Autodesk Inventor part; units mm, degrees
ref_plane "YZ Plane" through (0, 0, 0) normal (1, 0, 0) x (0, 1, 0)
ref_plane "XZ Plane" through (0, 0, 0) normal (0, 1, 0) x (-1, 0, 0)
ref_plane "XY Plane" through (0, 0, 0) normal (0, 0, 1) x (1, 0, 0)
sketch "Sketch1" plane through (0, 0, 0) normal (0, 1, 0) x (-1, 0, 0)
  line L0 (20.05, -10.07) -> (-20.05, -10.07)
  line L1 (-20.05, -10.07) -> (-20.05, 10.07)
  line L2 (-20.05, 10.07) -> (20.05, 10.07)
  line L3 (20.05, 10.07) -> (20.05, -10.07)
  point P0 (0, 0)
  point P1 (0, -10.07)
  point P2 (20.05, 0)
  dimension "d0" = 40.1
  dimension "d1" = 20.14
extrude "Extrusion1" add sketch "Sketch1" along normal blind 4
sketch "Sketch3" plane through (0, 0, 0) normal (0, -1, 0) x (1, 0, 0)
  ellipse E0 centre (-17.932, 7.952) end of major axis (-18.798, 8.818) minor radius 1 (-18.1556, 9.07) -> (-19.05, 8.1756) ccw
  line L0 (-19.05, -8.1756) -> (-19.05, 8.1756)
  ellipse E1 centre (-17.932, -7.952) end of major axis (-18.798, -8.818) minor radius 1 (-19.05, -8.1756) -> (-18.1556, -9.07) ccw
  line L1 (18.1556, -9.07) -> (-18.1556, -9.07)
  ellipse E2 centre (17.932, -7.952) end of major axis (18.798, -8.818) minor radius 1 (18.1556, -9.07) -> (19.05, -8.1756) ccw
  line L2 (19.05, 8.1756) -> (19.05, -8.1756)
  ellipse E3 centre (17.932, 7.952) end of major axis (18.798, 8.818) minor radius 1 (19.05, 8.1756) -> (18.1556, 9.07) ccw
  line L3 (-18.1556, 9.07) -> (18.1556, 9.07)
  circle A0 centre (17.55, -7.525) radius 0.7835
  circle A1 centre (17.55, 7.525) radius 0.7835
  circle A2 centre (2.45, -7.525) radius 0.7835
  circle A3 centre (2.45, 7.525) radius 0.7835
  circle A4 centre (-17.55, -7.525) radius 0.7835
  circle A5 centre (-17.55, 7.525) radius 0.7835
  circle A6 centre (-10.05, 0) radius 6.4
  circle A7 centre (-10.05, 0) radius 6.5
  point P0 (0, 0)
  dimension "d11" = 13
extrude "Extrusion2" cut sketch "Sketch3" against normal through all contours A6
sketch "Sketch7" plane through (0, 0, 0) normal (0, -1, 0) x (1, 0, 0)
  line L0 (16.15, -10.17) -> (-0.9759, -10.17)
  arc A0 (-0.9759, -10.17) -> (-0.9759, 10.17) centre (10.05, 0) ccw
  line L1 (-0.9759, 10.17) -> (16.15, 10.17)
  line L2 (16.15, 10.17) -> (16.15, 8.07)
  arc A1 (16.15, 8.07) -> (18.05, 6.17) centre (18.05, 8.07) ccw
  line L3 (18.05, 6.17) -> (20.15, 6.17)
  line L4 (20.15, 6.17) -> (20.15, -6.17)
  line L5 (20.15, -6.17) -> (18.05, -6.17)
  arc A2 (18.05, -6.17) -> (16.15, -8.07) centre (18.05, -8.07) ccw
  line L6 (16.15, -8.07) -> (16.15, -10.17)
  circle A3 centre (10.05, 0) radius 15.5
  circle A4 centre (-10.05, 0) radius 6.4
  circle A5 centre (-10.05, 0) radius 6.4
  point P0 (0, 0)
  point P1 (-4.9575, 3.8763)
  point P2 (-4.9575, -3.8763)
  dimension "d31" = 31
extrude "Extrusion4" add sketch "Sketch7" against normal up to surface (4 mm away) contours L6 A2 L5 L4 L3 A1 L2 L1 A0 L0 | A3 A4 picked at (9.8263, 0)
sketch "Sketch8" plane through (0, 4, 0) normal (0, 1, 0) x (1, 0, 0)
  circle A0 centre (10.05, 7) radius 0.7835
  circle A1 centre (17.05, 0) radius 0.7835
  circle A2 centre (10.05, -7) radius 0.7835
  circle A3 centre (3.05, 0) radius 0.7835
  circle A4 centre (10.05, 0) radius 1.75
  circle A5 centre (10.05, 0) radius 9.96
  point P0 (0, 0)
hole "Hole4" at (10.05, 4, 7) at (3.05, 4, 0) at (17.05, 4, 0) at (10.05, 4, -7) direction (0, -1, 0) diameter 2.1 end through all counterbore diameter 4.3 counterbore depth 1.5
sketch "Sketch9" plane through (0, 4, 0) normal (0, 1, 0) x (1, 0, 0)
  circle A0 centre (10.05, 0) radius 4.5
  circle A1 centre (10.05, 0) radius 2.925
  circle A2 centre (10.05, 0) radius 2.975
  point P0 (0, 0)
  dimension "d41" = 5.95
extrude "Extrusion5" cut sketch "Sketch9" against normal through all contours A1 | A2
sketch "Sketch10" plane through (0, 0, 0) normal (0, -1, 0) x (1, 0, 0)
  ellipse E0 centre (-17.932, 7.952) end of major axis (-18.798, 8.818) minor radius 1 (-18.1556, 9.07) -> (-19.05, 8.1756) ccw
  line L0 (-19.05, -8.1756) -> (-19.05, 8.1756)
  ellipse E1 centre (-17.932, -7.952) end of major axis (-18.798, -8.818) minor radius 1 (-19.05, -8.1756) -> (-18.1556, -9.07) ccw
  line L1 (18.1556, -9.07) -> (-18.1556, -9.07)
  ellipse E2 centre (17.932, -7.952) end of major axis (18.798, -8.818) minor radius 1 (18.1556, -9.07) -> (19.05, -8.1756) ccw
  line L2 (19.05, 8.1756) -> (19.05, -8.1756)
  ellipse E3 centre (17.932, 7.952) end of major axis (18.798, 8.818) minor radius 1 (19.05, 8.1756) -> (18.1556, 9.07) ccw
  line L3 (-18.1556, 9.07) -> (18.1556, 9.07)
  circle A0 centre (17.55, -7.525) radius 0.7835
  circle A1 centre (17.55, 7.525) radius 0.7835
  circle A2 centre (2.45, -7.525) radius 0.7835
  circle A3 centre (2.45, 7.525) radius 0.7835
  circle A4 centre (-17.55, -7.525) radius 0.7835
  circle A5 centre (-17.55, 7.525) radius 0.7835
  circle A6 centre (-10.05, 0) radius 6.4
  point P0 (0, 0)
hole "Hole5" at (17.55, 0, -7.525) at (2.45, 0, -7.525) at (-17.55, 0, -7.525) at (17.55, 0, 7.525) at (2.45, 0, 7.525) at (-17.55, 0, 7.525) direction (0, 1, 0) diameter 2.1 end through all counterbore diameter 4.3 counterbore depth 1.5
properties part number "gripper_6&7_connector" material "Aluminum 6061-AHC"
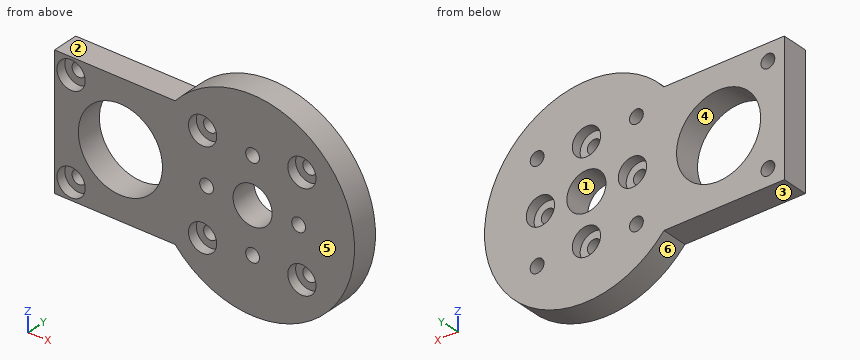
Design review of the part built by this model. Coordinates are the model's own, in mm. Face numbers are marked on the shaded views. A direction names the side the tool comes from. Round coordinates to 2 decimals unless told otherwise and drop trailing zeros. Write each loop counter-clockwise with the first axis right and the second up, starting at its lowest first coordinate (ties: lowest second). Pieces come first, ordered by that corner, then holes.
Item 1: For probe 1 along Z at (x, y) = (10.05, 2.95) (3 decimals); probe 2 along Z at (x, y) = (2.45, 0.95) (3 decimals); probe 3 along X at (y, z) = (3.15, 8), list the stretches that pass through material, from the lowest coordinate up.
Item 2: Clearance check with flat-ended pins moving along their axes: pin 1 Ø1.2 at (x, y) = (-8.5, 1.5) entering from -Z; pin 2 Ø2 at (x, z) = (9, 0) entering from +Y; pin 3 Ø2 at (x, z) = (1.5, 7.5) entering from -Y; pin 4 Ø1.3 at (x, z) = (10.5, -8) entering from +Y. State where each tip first meets the part, or that it passes through.
Item 3: We need section A-A on x = -17.55. Write out the cut boundary in (y, z) (3 decimals).
Item 4: We need section B-B on x = 17.55. Write out the cut boundary in (y, z) (3 decimals).
Item 5: The part is to be moulded in two halves that separate along X. For the marked faces 4, 5 and 6, say which applies: +X half, -X half, draft (parallel to the pull), parting line (faces both ways), or undercut.
Item 6: For the marked faces 1, 2 and 3, list the 3-axis set-ups (+Z, -Z, +X, -X, +Y, -Y) from which the entire face can be reached by the end or side of a thin tool; tool diameter is ignored.
Item 7: We need section D-D on z = 7.5. State how many separate pieces and enclosed holes the cut face has, and give its area (3 significant figures).
Item 8: We need section C-C on x = -8. Write out the cut boundary in (y, z), and give its area (3 significant figures).
Returned:
1. probe 1: z = -15.5 to -9.15, -4.85 to -2.975, 2.975 to 4.85, 9.15 to 15.5
1. probe 2: z = -13.509 to -9.675, -5.375 to -0.862, 0.862 to 5.375, 9.675 to 13.509
1. probe 3: x = -20.05 to -18.49, -16.61 to 1.51, 3.39 to 8.15, 11.95 to 16.61, 18.49 to 23.33
2. pin 1: stops at z = -10.07
2. pin 2: passes through
2. pin 3: stops at y = 1.5
2. pin 4: stops at y = 2.5
3. outline: (0, -10.07) - (4, -10.07) - (4, -8.575) - (1.5, -8.575) - (1.5, -9.675) - (0, -9.675) - close; (0, -5.375) - (1.5, -5.375) - (1.5, -6.475) - (4, -6.475) - (4, 6.475) - (1.5, 6.475) - (1.5, 5.375) - (0, 5.375) - close; (0, 9.675) - (1.5, 9.675) - (1.5, 8.575) - (4, 8.575) - (4, 10.07) - (0, 10.07) - close
4. outline: (0, -13.565) - (4, -13.565) - (4, -8.575) - (1.5, -8.575) - (1.5, -9.675) - (0, -9.675) - close; (0, -5.375) - (1.5, -5.375) - (1.5, -6.475) - (4, -6.475) - (4, -2.091) - (2.5, -2.091) - (2.5, -0.923) - (0, -0.923) - close; (0, 0.923) - (2.5, 0.923) - (2.5, 2.091) - (4, 2.091) - (4, 6.475) - (1.5, 6.475) - (1.5, 5.375) - (0, 5.375) - close; (0, 9.675) - (1.5, 9.675) - (1.5, 8.575) - (4, 8.575) - (4, 13.565) - (0, 13.565) - close
5. face 4: undercut
5. face 5: draft
5. face 6: parting line
6. face 1: +Y, -Y
6. face 2: +Z, -X, +Y, -Y
6. face 3: -Z, -X, +Y, -Y
7. separate pieces: 5
7. enclosed holes: 0
7. area: 129 mm2
8. outline: (0, -10.07) - (4, -10.07) - (4, -6.06) - (0, -6.06) - close; (0, 6.06) - (4, 6.06) - (4, 10.07) - (0, 10.07) - close
8. area: 32.1 mm2
